Source: three-view drawing plus pictorial views. Frame: mm from the lowest corner of the part. A direction names the side the tool comes from. Coordinates: 2 decimals unless noted, no trailing zeros. Write each loop counter-clockwise with the first axis right and the second up, starting at its lowest first coordinate (ties: lowest second). Pieces come first, ordered by that corner, then holes. Notation, with made-up numbers: (-11.5, 81.5) - (-0.5, 81.5) arc R32 cw to (-0.5, 114.5) - close; hole circle Ø10 at (72, 39). An arc over 180 degrees is marked (long way). Put each result on its own line as item: value.
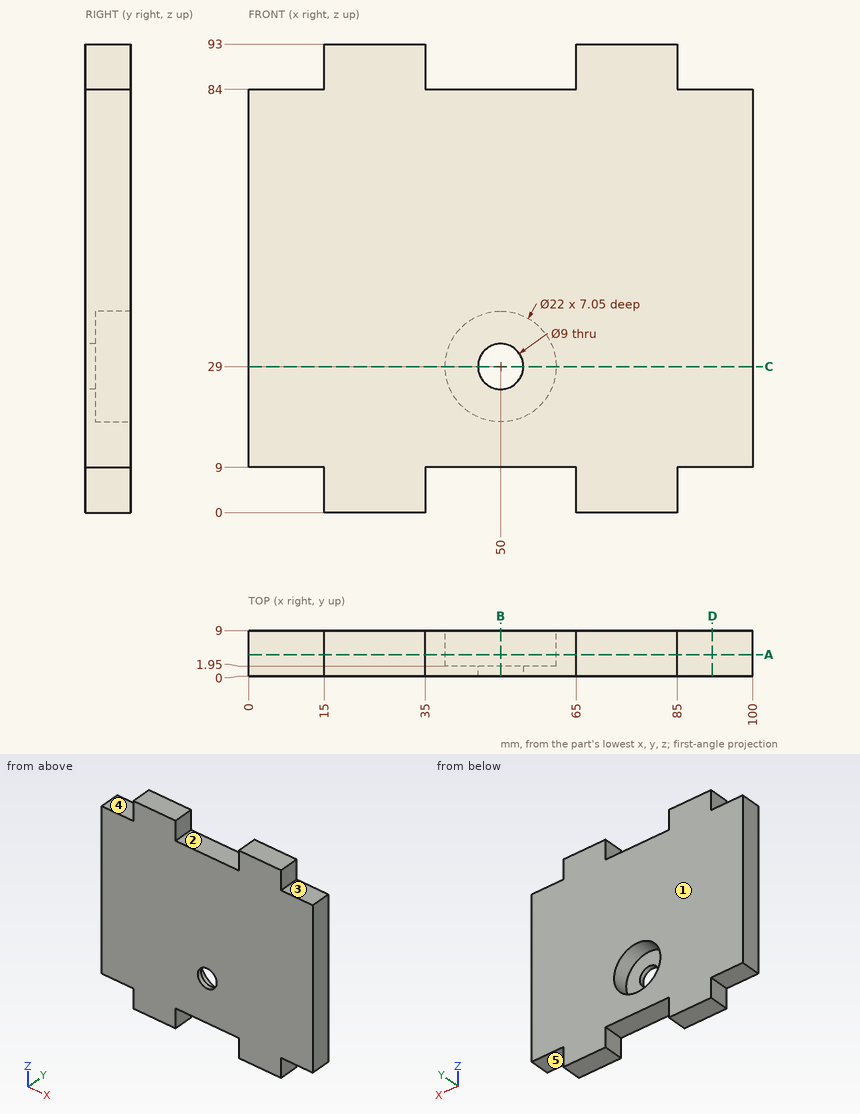
1. Ray query, probe 1 along Z at (x, y) = (50, 1.15); probe 2 along X at (y, z) = (1.4, 29); probe 3 along Z at (x, y) = (40, 8.75). Return the intervals inside material, ascending. Write a range as from..to.
Answer below:
probe 1: z = 9..24.5, 33.5..84
probe 2: x = 0..45.5, 54.5..100
probe 3: z = 9..24.42, 33.58..84
2. Section query C-C (z = 29). Return loops of the section in (x, y), then the cut area to 3 significant figures.
Answer below:
outline: (0, 0) - (45.5, 0) - (45.5, 1.95) - (39, 1.95) - (39, 9) - (0, 9) - close; (54.5, 0) - (100, 0) - (100, 9) - (61, 9) - (61, 1.95) - (54.5, 1.95) - close
area: 727 mm²
3. Section query A-A (y = 4.25). Return loops of the section in (x, z), then the cut area to 3 significant figures.
Answer below:
outline: (0, 9) - (15, 9) - (15, 0) - (35, 0) - (35, 9) - (65, 9) - (65, 0) - (85, 0) - (85, 9) - (100, 9) - (100, 84) - (85, 84) - (85, 93) - (65, 93) - (65, 84) - (35, 84) - (35, 93) - (15, 93) - (15, 84) - (0, 84) - close; hole circle Ø22 at (50, 29)
area: 7,840 mm²
4. Section query B-B (x = 50). Return loops of the section in (y, z).
Answer below:
outline: (0, 9) - (9, 9) - (9, 18) - (1.95, 18) - (1.95, 24.5) - (0, 24.5) - close; (0, 33.5) - (1.95, 33.5) - (1.95, 40) - (9, 40) - (9, 84) - (0, 84) - close
5. Mould query, pull axis X, two halves, no side actions, for the marked faces 1 and 2. Classes: +X half, -X half, draft (parallel to the pull), parting line (faces both ways), or undercut.
Answer below:
face 1: draft
face 2: undercut
6. Section query D-D (x = 92). Return loops of the section in (y, z), then the cut area to 3 significant figures.
Answer below:
outline: (0, 9) - (9, 9) - (9, 84) - (0, 84) - close
area: 675 mm²
7. Pin query (flat end, axial travel): pin 1 Ø4.5 at (y, z) = (6.5, 2.5) entering from -X; pin 2 Ø13 at (x, z) = (50, 29) entering from +Y; pin 3 Ø2.5 at (y, z) = (3.5, 2.5) entering from +X. Return the tip coordinate at first contact, or that it passes through.
Answer below:
pin 1: stops at x = 15
pin 2: stops at y = 1.95
pin 3: stops at x = 85
8. Set-up query: the marked faces 3, 4 and 5. Return all of +Z, -Z, +X, -X, +Y, -Y with unobstructed straight access to the full face (end or side cutting, diameter ignored); none if empty.
Answer below:
face 3: +Z, +X, +Y, -Y
face 4: +Z, -X, +Y, -Y
face 5: -Z, +X, +Y, -Y
